from build123d import *

# Parameters (mm, degrees)
F2_DEPTH              = 70
F3_R                  = 5.6
F4_R                  = 2.6
F5_W                  = 70
F5_H                  = 3
F5_W_2                = 3
F5_H_2                = 70
F6_DEPTH              = 35
F7_R                  = 5
F10_D                 = 10.2
F10_CBORE_D           = 17
F10_CBORE_DEPTH       = 1.5
F10_ON_F9_D           = 10.2
F10_ON_F9_CBORE_D     = 17
F10_ON_F9_CBORE_DEPTH = 1.5


with BuildPart() as f2:
    # F1 (on Front) → F2 (new body)
    with BuildSketch(Plane.XZ):
        Polygon((3, 196), (0, 196), (0, 0), (196, 0), (196, 3), (3, 3), align=None)
    extrude(amount=-F2_DEPTH)

    # F3
    f3_edges = [f2.edges().sort_by_distance(p)[0] for p in [
        (0, 35, 0),
    ]]
    fillet(f3_edges, radius=F3_R)

    # F4
    f4_edges = [f2.edges().sort_by_distance(p)[0] for p in [
        (3, 35, 3),
    ]]
    fillet(f4_edges, radius=F4_R)

    # F5 (on face) → F6 (join)
    with BuildSketch(Plane.XZ):
        with Locations((51, 1.5)):
            Rectangle(F5_W, F5_H)
        with Locations((1.5, 51)):
            Rectangle(F5_W_2, F5_H_2)
    extrude(amount=F6_DEPTH)

    # F7
    f7_edges = [f2.edges().sort_by_distance(p)[0] for p in [
        (16, 0, 1.5),
        (16, -35, 1.5),
        (86, -35, 1.5),
        (86, 0, 1.5),
        (1.5, -35, 16),
        (1.5, -35, 86),
        (1.5, 0, 16),
        (1.5, 0, 86),
        (1.5, 0, 196),
        (1.5, 70, 196),
        (196, 70, 1.5),
        (196, 0, 1.5),
    ]]
    fillet(f7_edges, radius=F7_R)

    # F10 (through all)
    with Locations(Plane(origin=(0, 0, 0), x_dir=(1, 0, 0), z_dir=(0, 0, -1))):
        with Locations((38, -35), (108, -35), (178, -35)):
            CounterBoreHole(F10_D / 2, F10_CBORE_D / 2, F10_CBORE_DEPTH)

    # F10 on F9 (through all)
    with Locations(Plane(origin=(0, 0, 0), x_dir=(0, -1, 0), z_dir=(-1, 0, 0))):
        with Locations((-35, 178), (-35, 108), (-35, 38)):
            CounterBoreHole(F10_ON_F9_D / 2, F10_ON_F9_CBORE_D / 2, F10_ON_F9_CBORE_DEPTH)


solid = f2.part
Geometry check sheet. Reference: the model listing, model coordinates, mm. A direction names the side the tool comes from. Round coordinates to 2 decimals unless told otherwise and drop trailing zeros. Write each loop counter-clockwise with the first axis right and the second up, starting at its lowest first coordinate (ties: lowest second). Pieces come first, ordered by that corner, then holes.
Item 1: Section check A-A (z = 38). Record the boundary of the cut face in (x, y), plus the area to 3 significant figures.
Determined:
outline: (0, -35) - (3, -35) - (3, 29.9) - (1.5, 29.9) - (1.5, 26.5) - (0, 26.5) - close; (0, 43.5) - (1.5, 43.5) - (1.5, 40.1) - (3, 40.1) - (3, 70) - (0, 70) - close
area: 274 mm2
Item 2: Material ranges on line 1 along X through (y, z) = (35, 2); line 2 along Y through (x, z) = (38, 2); line 3 along Z through (x, y) = (0.7, 35), recorded low to high.
Determined:
line 1: x = 1.31 to 32.9, 43.1 to 102.9, 113.1 to 172.9, 183.1 to 196
line 2: y = -35 to 29.9, 40.1 to 70
line 3: z = 2.89 to 29.5, 46.5 to 99.5, 116.5 to 169.5, 186.5 to 196
Item 3: Go/stop test with flat-tipped pins: pin 1 Ø8 at (x, y) = (178, 35) entering from +Z; pin 2 Ø19.5 at (y, z) = (35, 38) entering from +X; pin 3 Ø3.5 at (y, z) = (-13.5, 1) entering from -X; pin 4 Ø3.5 at (x, z) = (142, 1.5) entering from -Y. Record where each tip stops, or that it passes through.
Determined:
pin 1: passes through
pin 2: stops at x = 3
pin 3: stops at x = 16
pin 4: stops at y = 0
Item 4: Section check D-D (y = 21.5). Record the boundary of the cut face in (x, z), plus the area to 3 significant figures.
Determined:
outline: (0, 5.6) arc R5.6 ccw to (5.6, 0) - (196, 0) - (196, 3) - (5.6, 3) arc R2.6 cw to (3, 5.6) - (3, 196) - (0, 196) - close
area: 1,160 mm2
Item 5: Mould release check, pull along Z, two halves, no side actions. Record for faces 4 (the face through (106.16, 43.3, 0.74)), 5 (the face through (1.5, 31, 174)), 6 (the face through (2, -1, 14)): +Z half, -Z half, draft (parallel to the pull), parting line (faces both ways), or undercut.
Determined:
face 4: draft
face 5: undercut
face 6: -Z half
Item 6: Access from +Z, -Z, +X, -X, +Y, -Y to the whole of each face (thin tool, end or side, straight path). Record for faces 1 (the face through (2.3, 31.2, 181.4)), 2 (the face through (0.74, 36.84, 99.7)), 3 (the face through (112, 39, 1.5)).
Determined:
face 1: +X, -X
face 2: -X
face 3: -Z
Item 7: Section check B-B (x = 178). Record the boundary of the cut face in (y, z), plus the area to 3 significant figures.
Determined:
outline: (0, 0) - (26.5, 0) - (26.5, 1.5) - (29.9, 1.5) - (29.9, 3) - (0, 3) - close; (40.1, 1.5) - (43.5, 1.5) - (43.5, 0) - (70, 0) - (70, 3) - (40.1, 3) - close
area: 169 mm2
Item 8: Section check C-C (y = -10). Record the boundary of the cut face in (x, z), plus the area to 3 significant figures.
Determined:
outline: (0, 16) - (3, 16) - (3, 86) - (0, 86) - close; (16, 0) - (86, 0) - (86, 3) - (16, 3) - close
area: 420 mm2
